Geometry: see drawing. Coordinates: mm, zero at the bounding-box minimum. Give positions to 0.01 mm unless a question says otherwise; leave off trailing zeros. Order: outer loops, then holes, each group sorted by start corner. A loop starts at its lowest first (then second) coordinate and runs counter-clockwise, first axis right, second up. Notation, with made-up numbers: (70.5, 62.25) - (118.5, 62.25) arc R29 ccw to (118.5, 90.25) - close; hole circle Ø2 at (-23, -39). An arc over 180 degrees is marked (long way). Put each result on its own line as item: value. Start each with the question number.
1. Mould query, pull axis Y, two halves, no side actions, for the marked faces 1, 2 and 3. Classes: pulls with the +Y half, pulls with the -Y half, needs draft (parallel to the pull), parting line crosses it, or undercut.
2. Section C-C on y = 3. Return the cut outline in (x, z), plus the area to 3 significant figures.
3. Section D-D on x = 9.75. Return the cut outline in (y, z).
4. Ray query, line 1 along X through (y, z) = (3.5, 12.75); line 2 along Y through (x, z) = (12.75, 3); line 3 along Z through (x, y) = (14.75, 5.5). Return the intervals inside material, ascending. Write a range as from..to.
5. Section B-B on z = 12.75. Return the cut outline in (x, y).
6. Section A-A on x = 12.75. Return the cut outline in (y, z).
7. First-contact query: P1, Ø3, axis at y = 5, z = 17.5, coming from the -X side; P2, Ø2, axis at y = 3.5, z = 16.5, coming from the -X side. Flat tips, straight axial feed; report the tip coordinate or a pass-through.
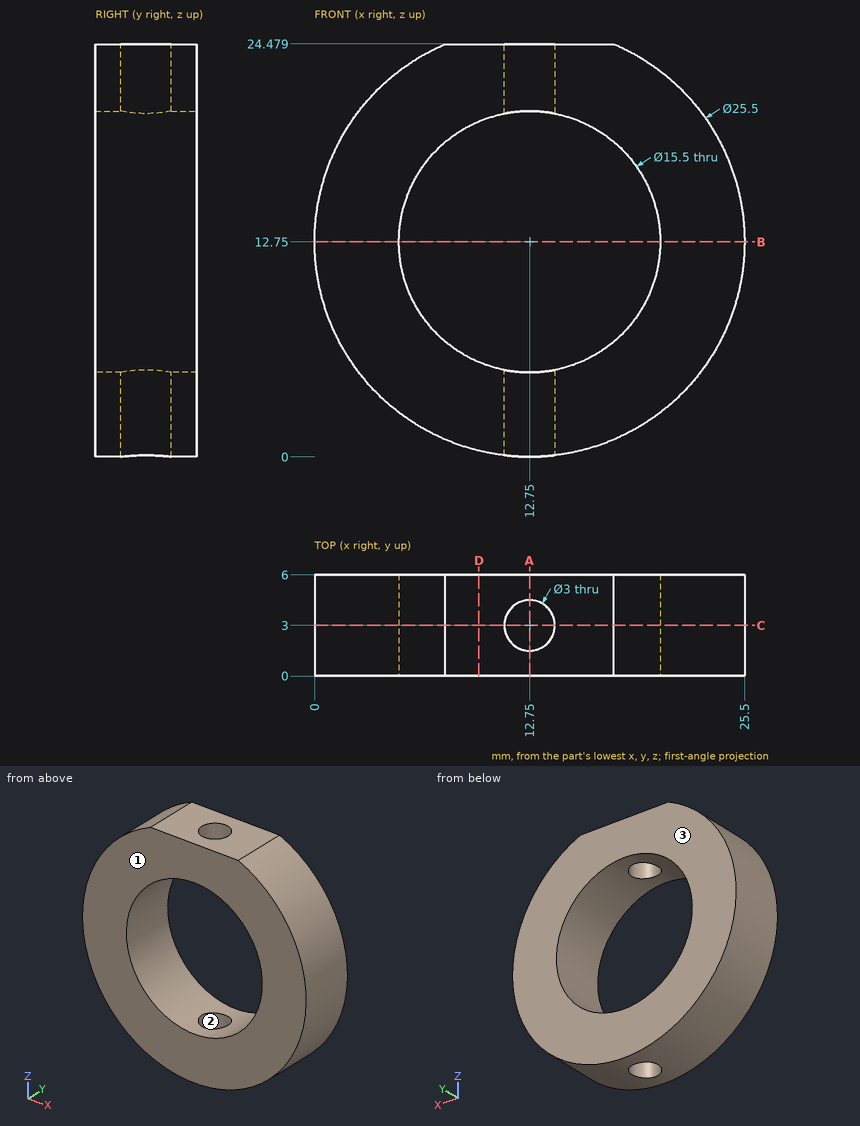
Resolved:
1. face 1: pulls with the -Y half
1. face 2: undercut
1. face 3: pulls with the +Y half
2. outline: (7.75, 24.48) arc R12.75 ccw to (11.25, 0.09) - (11.25, 5.15) arc R7.75 cw to (11.25, 20.35) - (11.25, 24.48) - close; (14.25, 0.09) arc R12.75 ccw to (17.75, 24.48) - (14.25, 24.48) - (14.25, 20.35) arc R7.75 cw to (14.25, 5.15) - close
2. area: 288 mm^2
3. outline: (0, 0.36) - (6, 0.36) - (6, 5.6) - (0, 5.6) - close; (0, 19.9) - (6, 19.9) - (6, 24.48) - (0, 24.48) - close
4. line 1: 0..5, 20.5..25.5
4. line 2: 0..1.5, 4.5..6
4. line 3: 0.16..5.26, 20.24..24.48
5. outline: (0, 0) - (5, 0) - (5, 6) - (0, 6) - close; (20.5, 0) - (25.5, 0) - (25.5, 6) - (20.5, 6) - close
6. outline: (0, 0) - (1.5, 0) - (1.5, 5) - (0, 5) - close; (0, 20.5) - (1.5, 20.5) - (1.5, 24.48) - (0, 24.48) - close; (4.5, 0) - (6, 0) - (6, 5) - (4.5, 5) - close; (4.5, 20.5) - (6, 20.5) - (6, 24.48) - (4.5, 24.48) - close
7. P1: x = 0.42
7. P2: x = 0.3
